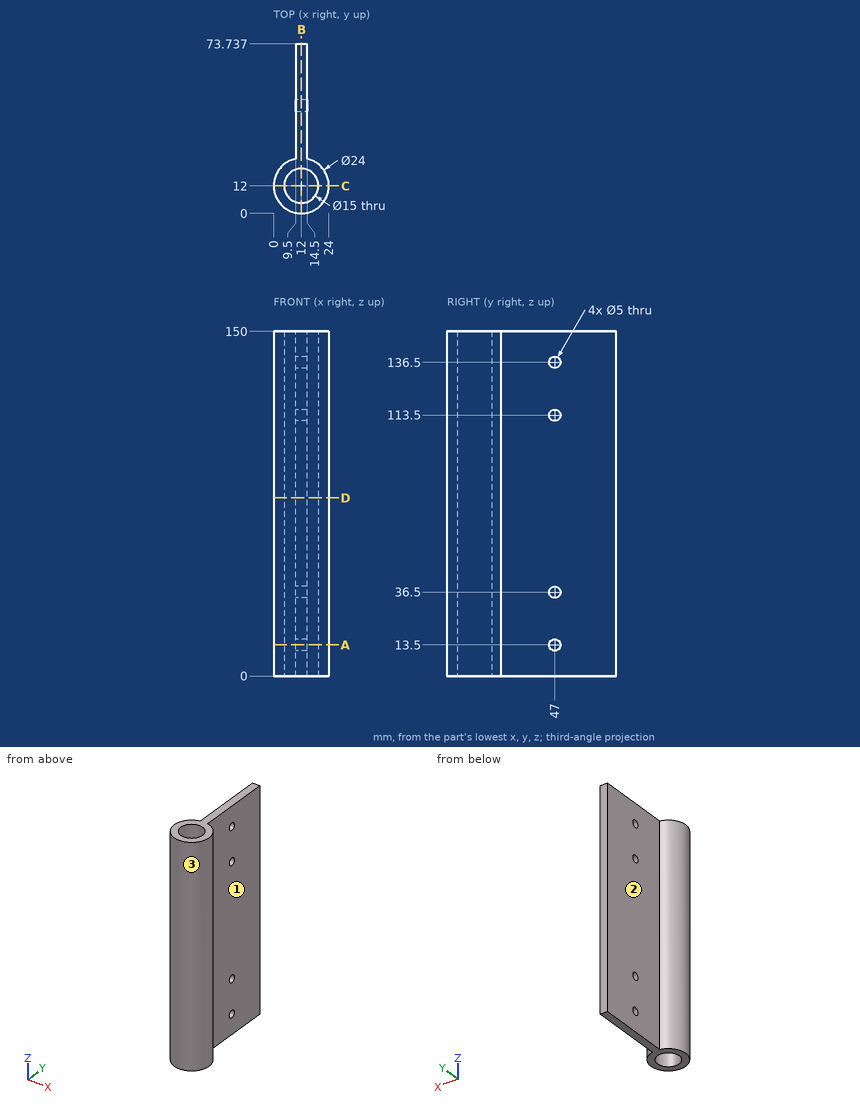
Answer from the drawing. Dimensions are ordinates in mm from the lowest x, y and z of the part. A direction names the side the tool comes from. Round coordinates to 2 decimals unless told otherwise and drop trailing zeros. Write each loop counter-clockwise with the first axis right and the second up, starting at its lowest first coordinate (ties: lowest second). Pieces come first, ordered by that corner, then holes.
1. The part is cut by section D-D, the plane z = 77.5. Determine the outline of the cut face in (x, y), then the cut area to 3 significant figures.
2. Straight lines are drawn through the part: L1, parallel to Z at x = 11.9, y = 47; L2, parallel to X at y = 12.5, z = 17.5; L3, parallel to X at y = 31, z = 7. For each, find the intervals that lie inside material, in ascending order.
3. The part is cut by section C-C, the plane y = 12. Determine the outline of the cut face in (x, z).
4. Which of the six approach directions +Z, -Z, +X, -X, +Y, -Y give full straight-line access (tool end or side, diameter ignored) to the marked faces 1, 2 and 3?
5. The part is cut by section A-A, the plane z = 13.5. Determine the outline of the cut face in (x, y).
6. The part is cut by section B-B, the plane x = 12. Determine the outline of the cut face in (y, z), then the cut area to 3 significant figures.
7. Given pin 1 Ø1.5 at (y, z) = (49.5, 38.5) entering from +X; pin 2 Ø5 at (x, z) = (3.5, 113.5) entering from +Y; pin 3 Ø9 at (x, y) = (12, 12) entering from -Z; pin 4 Ø8 at (y, z) = (47, 13.5) entering from -X, each flat-ended and moving along its own axis, determine where each tip first touches the part or whether it passes through.
Values:
1. outline: (9.5, 23.74) arc R12 ccw (long way) to (14.5, 23.74) - (14.5, 73.74) - (9.5, 73.74) - close; hole circle Ø15 at (12, 12)
1. area: 525 mm2
2. L1: z = 0 to 11, 16 to 34, 39 to 111, 116 to 134, 139 to 150
2. L2: x = 0.01 to 4.52, 19.48 to 23.99
2. L3: x = 9.5 to 14.5
3. outline: (0, 0) - (4.5, 0) - (4.5, 150) - (0, 150) - close; (19.5, 0) - (24, 0) - (24, 150) - (19.5, 150) - close
4. face 1: +Z, -Z, +X, +Y
4. face 2: +Z, -Z, -X, +Y
4. face 3: +Z, -Z
5. outline: (9.5, 23.74) arc R12 ccw (long way) to (14.5, 23.74) - (14.5, 44.5) - (9.5, 44.5) - close; (9.5, 49.5) - (14.5, 49.5) - (14.5, 73.74) - (9.5, 73.74) - close; hole circle Ø15 at (12, 12)
6. outline: (0, 0) - (4.5, 0) - (4.5, 150) - (0, 150) - close; (19.5, 0) - (73.74, 0) - (73.74, 150) - (19.5, 150) - close; hole circle Ø5 at (47, 13.5); hole circle Ø5 at (47, 36.5); hole circle Ø5 at (47, 113.5); hole circle Ø5 at (47, 136.5)
6. area: 8,730 mm2
7. pin 1: stops at x = 14.5
7. pin 2: stops at y = 22.39
7. pin 3: passes through
7. pin 4: stops at x = 9.5
